```python
from build123d import *

# Parameters (mm, degrees)
F0_R     = 50.8
F0_R_2   = 3.175
F0_R_3   = 38.1
F1_DEPTH = 25.4


# Not quite as in the source:
# - a fillet or chamfer that OpenCascade refuses, or shapes differently, is made with other operations: its cross-section is extruded or revolved along the edge and cut away or added


with BuildPart() as f1:
    # F0 (on Front) → F1 (new body)
    with BuildSketch(Plane.XZ):
        Circle(F0_R)
        with Locations((-44.45, 0)):
            Circle(F0_R_2, mode=Mode.SUBTRACT)
        Circle(F0_R_3, mode=Mode.SUBTRACT)
        with Locations((22.225, -38.4948291982)):
            Circle(F0_R_2, mode=Mode.SUBTRACT)
        with Locations((22.225, 38.4948291982)):
            Circle(F0_R_2, mode=Mode.SUBTRACT)
    extrude(amount=F1_DEPTH)

    # F2: fillet of radius 5.08 on 4 edges, made by hand

    # F2_s1 → F2_t2 (revolve, cut)
    with BuildSketch(Plane.XY):
        with BuildLine():
            ThreePointArc((50.8, -5.08), (49.3121024484, -1.4878975516), (45.72, 0))
            Line((45.72, 0), (50.8, 0))
            Line((50.8, 0), (50.8, -5.08))
        make_face()
    revolve(axis=Axis((0, 0, 0), (0, -1, 0)), mode=Mode.SUBTRACT)

    # F2_s3 → F2_t4 (revolve, cut)
    with BuildSketch(Plane.XY):
        with BuildLine():
            ThreePointArc((38.1, -5.08), (39.5878975516, -1.4878975516), (43.18, 0))
            Line((43.18, 0), (38.1, 0))
            Line((38.1, 0), (38.1, -5.08))
        make_face()
    revolve(axis=Axis((0, 0, 0), (0, -1, 0)), mode=Mode.SUBTRACT)

    # F2_s5 → F2_t6 (revolve, cut)
    with BuildSketch(Plane.XY):
        with BuildLine():
            ThreePointArc((38.1, -20.32), (39.5878975516, -23.9121024484), (43.18, -25.4))
            Line((43.18, -25.4), (38.1, -25.4))
            Line((38.1, -25.4), (38.1, -20.32))
        make_face()
    revolve(axis=Axis((0, -25.4, 0), (0, -1, 0)), mode=Mode.SUBTRACT)

    # F2_s7 → F2_t8 (revolve, cut)
    with BuildSketch(Plane.XY):
        with BuildLine():
            ThreePointArc((50.8, -20.32), (49.3121024484, -23.9121024484), (45.72, -25.4))
            Line((45.72, -25.4), (50.8, -25.4))
            Line((50.8, -25.4), (50.8, -20.32))
        make_face()
    revolve(axis=Axis((0, -25.4, 0), (0, -1, 0)), mode=Mode.SUBTRACT)


solid = f1.part
```
Check sheet for the modelled part. Datum: model origin and axes. Units: mm. Round coordinates to 2 decimals unless told otherwise and drop trailing zeros. Order: outer loops, then holes, each group sorted by start corner. A loop starts at its lowest first (then second) coordinate and runs counter-clockwise, first axis right, second up. Notation, with made-up numbers: M 4.25,76 L 53.25,76 A20 cw 53.25,91 Z; hole C -16.75,-38 d8. An arc over 180 degrees is marked long. Answer in a Markdown table with one row per item.
(1) Section check B-B on z = 0. Record the boundary of the cut face in (x, y) (3 decimals).
Findings:
| item | result |
|---|---|
| outline | M -50.8,-20.32 A5.08 ccw -47.625,-25.029 L -47.625,-0.371 A5.08 ccw -50.8,-5.08 Z; M -41.275,-25.029 A5.08 ccw -38.1,-20.32 L -38.1,-5.08 A5.08 ccw -41.275,-0.371 Z; M 38.1,-20.32 A5.08 ccw 43.18,-25.4 L 45.72,-25.4 A5.08 ccw 50.8,-20.32 L 50.8,-5.08 A5.08 ccw 45.72,0 L 43.18,0 A5.08 ccw 38.1,-5.08 Z |
(2) Gauge pin test, flat ends, axial feed: pin 1 (8 mm diameter, centred on y = -15.5, z = -8.5, fed in from -X); pin 2 (4 mm diameter, centred on x = -44.45, z = 0, fed in from -Y); pin 3 (10 mm diameter, centred on x = 22.22, z = -38.49, fed in from +Y); pin 4 (1.5 mm diameter, centred on y = -16, z = -21.5, fed in from -X). Record the tip position at first contact, or that the pin passes through.
Findings:
| item | result |
|---|---|
| pin 1 | stops at x = -50.6 |
| pin 2 | passes through |
| pin 3 | stops at y = 0 |
| pin 4 | stops at x = -46.37 |
(3) Section check C-C on y = -13. Record the boundary of the cut face in (x, z) (3 decimals).
Findings:
| item | result |
|---|---|
| outline | C 0,0 d101.6; hole C -44.45,0 d6.35; hole C 0,0 d76.2; hole C 22.225,-38.495 d6.35; hole C 22.225,38.495 d6.35 |
(4) Section check D-D on y = -2.5. Record the boundary of the cut face in (x, z) (3 decimals), plus the area to 3 significant figures.
Findings:
| item | result |
|---|---|
| outline | C 0,0 d100.192; hole C -44.45,0 d6.35; hole C 0,0 d77.608; hole C 22.225,-38.495 d6.35; hole C 22.225,38.495 d6.35 |
| area | 3,060 mm^2 |
(5) Section check A-A on x = 0. Record the boundary of the cut face in (y, z), plus the area to 3 significant figures.
Findings:
| item | result |
|---|---|
| outline | M -25.4,-45.72 A5.08 ccw -20.32,-50.8 L -5.08,-50.8 A5.08 ccw 0,-45.72 L 0,-43.18 A5.08 ccw -5.08,-38.1 L -20.32,-38.1 A5.08 ccw -25.4,-43.18 Z; M -25.4,43.18 A5.08 ccw -20.32,38.1 L -5.08,38.1 A5.08 ccw 0,43.18 L 0,45.72 A5.08 ccw -5.08,50.8 L -20.32,50.8 A5.08 ccw -25.4,45.72 Z |
| area | 601 mm^2 |
(6) Draft check along X on faces 1 (the cylindrical face through (23.69, -12.52, -41.31)), 2 (the flat face through (-23, -25.4, -37)), 3 (the cylindrical face through (-11.012, -12.593, -49.592)). Enter one of: +X half, -X half, draft (parallel to the pull), parting line (faces both ways), or undercut.
Findings:
| item | result |
|---|---|
| face 1 | undercut |
| face 2 | draft |
| face 3 | parting line |
(7) Material ranges on line 1 along Z through (x, y) = (0, -12.75); line 2 along Z through (x, y) = (20.5, -18.75); line 3 along Z through (x, y) = (16, -12.5), recorded low to high. Write a range as from..to.
Findings:
| item | result |
|---|---|
| line 1 | z = -50.8..-38.1, 38.1..50.8 |
| line 2 | z = -46.48..-41.16, -35.83..-32.11, 32.11..35.83, 41.16..46.48 |
| line 3 | z = -48.21..-34.58, 34.58..48.21 |
